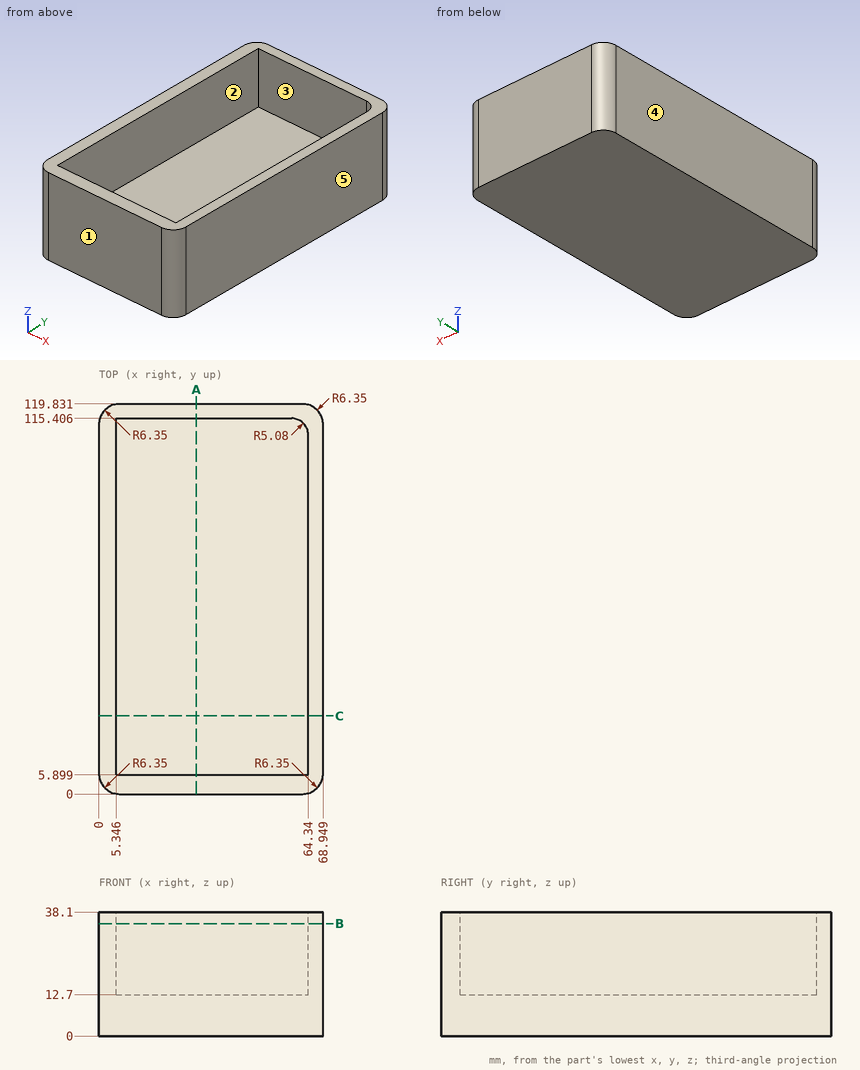
Could you check a few things on this drawing? It's one solid part, dimensions in mm from its lowest x, y, z. A direction names the side the tool comes from. Coordinates: 2 decimals unless noted, no trailing zeros. Write each loop counter-clockwise with the first axis right and the second up, starting at its lowest first coordinate (ties: lowest second). Pieces come first, ordered by that corner, then holes.
1) If we section it at A-A (x = 30): List the corners of the cut face in (y, z) for me, plus the area to 3 significant figures.
Filled in:
outline: (0, 0) - (119.83, 0) - (119.83, 38.1) - (115.41, 38.1) - (115.41, 12.7) - (5.9, 12.7) - (5.9, 38.1) - (0, 38.1) - close
area: 1,780 mm2
2) Which directions (+Z, -Z, +X, -X, +Y, -Y) give clear straight access to the entire face, cutting with the end or side of a thin tool? Please do the marked faces 1 and 2.
Filled in:
face 1: +Z, -Z, +X, -X, -Y
face 2: +Z
3) If I drill on line 1 (X direction, y = 80, z = 33); line 2 (Y direction, x = 43.5, z = 20.5); line 3 (Z direction, x = 55.5, y = 27.5), over which ranges is the centre line in solid material (lowest first)?
Filled in:
line 1: x = 0 to 5.35, 64.34 to 68.95
line 2: y = 0 to 5.9, 115.41 to 119.83
line 3: z = 0 to 12.7
4) Thinking about a two-plate mould opening in X: for the marked faces 3, 4 and 5, which applies, +X half, -X half, draft (parallel to the pull), parting line (faces both ways), or undercut?
Filled in:
face 3: undercut
face 4: -X half
face 5: +X half
5) I'm going to push flat-ended pins straight in: pin 1 (3 mm diameter, centred on x = 25, y = 31.5, fed in from +Z); pin 2 (2 mm diameter, centred on x = 47, y = 95.5, fed in from -Z). Where does each tip first touch, or does it pass through?
Filled in:
pin 1: stops at z = 12.7
pin 2: stops at z = 0
6) If we section it at B-B (z = 34.5): List the corners of the cut face in (x, y) for me, plus the area to 3 significant figures.
Filled in:
outline: (0, 6.35) arc R6.35 ccw to (6.35, 0) - (62.6, 0) arc R6.35 ccw to (68.95, 6.35) - (68.95, 113.48) arc R6.35 ccw to (62.6, 119.83) - (6.35, 119.83) arc R6.35 ccw to (0, 113.48) - close; hole (5.35, 5.9) - (64.34, 5.9) - (64.34, 110.33) arc R5.08 ccw to (59.26, 115.41) - (5.35, 115.41) - close
area: 1,770 mm2
7) If we section it at C-C (y = 24): List the corners of the cut face in (x, z) for me.
Filled in:
outline: (0, 0) - (68.95, 0) - (68.95, 38.1) - (64.34, 38.1) - (64.34, 12.7) - (5.35, 12.7) - (5.35, 38.1) - (0, 38.1) - close
